CAD build for the part. Positions are in the model's coordinates, mm. A direction names the side the tool comes from. Coordinates: 2 decimals unless noted, no trailing zeros. Write each loop counter-clockwise with the first axis right and the second up, starting at its lowest first coordinate (ties: lowest second). Pieces come first, ordered by that corner, then holes. Notation, with made-up numbers: (-3.5, 7.25) -> (0.5, 7.25) arc R19 ccw to (0.5, 37.25) -> close; hole circle Ø2 at (31, 54.25). An arc over 180 degrees is marked (long way). Answer as CSV lines item,"result".
```python
from build123d import *

# Parameters (mm, degrees)
SKETCH_2_R          = 1.61
CUT_EXTRUDE_1_DEPTH = 14.107106781
CHAMFER_1_SIZE      = 0.39
CHAMFER_2_SIZE      = 1


with BuildPart() as part:
    # Эскиз1 → Повернуть1 (revolve)
    with BuildSketch(Plane.XY):
        Polygon((0, 0), (14, 0), (14, -5), (5, -5), (5, -10), (4, -10), (4, -11.2), (5.2, -12.4), (4.492893219, -13.107106781), (2.585786438, -11.2), (2.585786438, -10), (0, -10), align=None)
    revolve(axis=Axis((0, -10, 0), (0, 1, 0)))

    # Эскиз2 → Вырез-Вытянуть1 (cut, through all)
    with BuildSketch(Plane(origin=(0, 0, 0), x_dir=(1, 0, 0), z_dir=(0, 1, 0))):
        Circle(SKETCH_2_R)
    extrude(amount=-CUT_EXTRUDE_1_DEPTH, mode=Mode.SUBTRACT)

    # Фаска1
    chamfer_1_edges = [part.edges().sort_by_distance(p)[0] for p in [
        (-1.61, -10, 0),
    ]]
    chamfer(chamfer_1_edges, length=CHAMFER_1_SIZE)

    # Фаска2
    chamfer_2_edges = [part.edges().sort_by_distance(p)[0] for p in [
        (-14, -5, 0),
        (-14, 0, 0),
    ]]
    chamfer(chamfer_2_edges, length=CHAMFER_2_SIZE)


solid = part.part
```
Item 1: Saw through at C-C on y = -2.5. Give the cut face in (x, z), and give its area (3 significant figures).
Answer below:
outline,"circle Ø28 at (0, 0); hole circle Ø3.22 at (0, 0)"
area,"608 mm2"
Item 2: Two-plate mould, pull along Y, no slides. Class faces 3 (the cylindrical face through (-2.583, -10.592, -0.114)), 4 (the flat face through (1, -10, 2)), 5 (the cylindrical face through (-0.867, -10.608, 3.905)): pulls with the +Y half, pulls with the -Y half, needs draft (parallel to the pull), parting line crosses it, or undercut.
Answer below:
face 3,"needs draft"
face 4,"pulls with the -Y half"
face 5,"undercut"
Item 3: Saw through at D-D on y = -5.5. Give the cut face in (x, z), and give its area (3 significant figures).
Answer below:
outline,"circle Ø10 at (0, 0); hole circle Ø3.22 at (0, 0)"
area,"70.4 mm2"
Item 4: 3-axis set-ups, long thin cutter, end or side, ignore diameter. For faces 1 (the cylindrical face through (-1.08, -7.54, 4.88)), 2 (the cylindrical face through (12.932, -2.521, 5.362)): which of +Z, -Z, +X, -X, +Y, -Y reach the whole face in a straight line?
Answer below:
face 1,"none"
face 2,"+Y, -Y"
Item 5: Flat gauge pins, fed straight in: pin 1 (1.6 mm diameter, centred on x = 1, z = -1, fed in from -Y); pin 2 (1.5 mm diameter, centred on x = 10.5, y = -2.5, fed in from -Z); pin 3 (5 mm diameter, centred on x = 6, y = -10, fed in from -Z). Where does each tip first touch, or does it go through?
Answer below:
pin 1,"stops at y = -10"
pin 2,"stops at z = -10.05"
pin 3,"stops at z = -3.57"
Item 6: Wall check: line 1 (X direction, y = -10.7, z = 0); line 2 (Z direction, x = 0, y = -3.25). Give the ranges that are in metal, low to high. Write a range as from..to.
Answer below:
line 1,"x = -4..-2.59, 2.59..4"
line 2,"z = -14..-1.61, 1.61..14"
